```python
from build123d import *

# Parameters (mm, degrees)
SKETCH1_W               = 100
SKETCH1_H               = 65
BOSS_EXTRUDE1_DEPTH     = 75
SKETCH5_W               = 41
SKETCH5_H               = 10
CUT_EXTRUDE1_DEPTH      = 141
SKETCH6_OUTSIDE_W       = 130.178
SKETCH6_OUTSIDE_H       = 95.178
SKETCH6_OUTSIDE_W_2     = 100
SKETCH6_OUTSIDE_H_2     = 40
CUT_EXTRUDE2_DEPTH      = 1
CUT_EXTRUDE2_DEPTH_BACK = 50
SKETCH7_W               = 50
SKETCH7_H               = 20
CUT_EXTRUDE3_DEPTH      = 40
SKETCH10_W              = 40
SKETCH10_H              = 25
CUT_EXTRUDE4_DEPTH      = 40


with BuildPart() as part:
    # Sketch1 → Boss-Extrude1 (new body)
    with BuildSketch(Plane(origin=(0, 0, 0), x_dir=(1, 0, 0), z_dir=(0, 1, 0))):
        with Locations((-6.156156156, 9.992492492)):
            Rectangle(SKETCH1_W, SKETCH1_H)
    extrude(amount=BOSS_EXTRUDE1_DEPTH)

    # Sketch5 → Cut-Extrude1 (cut)
    with BuildSketch(Plane(origin=(43.843843844, 0, 0), x_dir=(0, 0, -1), z_dir=(1, 0, 0))):
        with Locations((9.992492492, 5)):
            Rectangle(SKETCH5_W, SKETCH5_H)
    extrude(amount=-CUT_EXTRUDE1_DEPTH, mode=Mode.SUBTRACT)

    # Sketch6 outside → Cut-Extrude2 (cut, two sides)
    with BuildSketch(Plane(origin=(0, 75, 0), x_dir=(1, 0, 0), z_dir=(0, 1, 0))) as cut_extrude2_sk:
        with Locations((-6.156, 9.992)):
            Rectangle(SKETCH6_OUTSIDE_W, SKETCH6_OUTSIDE_H)
        with Locations((-6.156156156, 22.492492492)):
            Rectangle(SKETCH6_OUTSIDE_W_2, SKETCH6_OUTSIDE_H_2, mode=Mode.SUBTRACT)
    extrude(amount=CUT_EXTRUDE2_DEPTH, mode=Mode.SUBTRACT)
    extrude(cut_extrude2_sk.sketch, amount=-CUT_EXTRUDE2_DEPTH_BACK, mode=Mode.SUBTRACT)

    # Sketch7 → Cut-Extrude3 (cut)
    with BuildSketch(Plane(origin=(0, 75, 0), x_dir=(1, 0, 0), z_dir=(0, 1, 0))):
        with Locations((-6.156156156, 12.492492492)):
            Rectangle(SKETCH7_W, SKETCH7_H)
    extrude(amount=-CUT_EXTRUDE3_DEPTH, mode=Mode.SUBTRACT)

    # Sketch10 → Cut-Extrude4 (cut)
    with BuildSketch(Plane(origin=(0, 25, 0), x_dir=(1, 0, 0), z_dir=(0, 1, 0))):
        with Locations((-6.156156156, -10.007507508)):
            Rectangle(SKETCH10_W, SKETCH10_H)
    extrude(amount=-CUT_EXTRUDE4_DEPTH, mode=Mode.SUBTRACT)


solid = part.part
```
The listing builds one solid part. Answer for the finished solid, in the listing's coordinates (mm). A direction names the side the tool comes from. Give positions to 0.01 mm unless a question says otherwise; leave off trailing zeros. Order: outer loops, then holes, each group sorted by start corner. A loop starts at its lowest first (then second) coordinate and runs counter-clockwise, first axis right, second up. Notation, with made-up numbers: M 78.25,-6 L 125.25,-6 A33 cw 125.25,28 Z; hole C -33.5,-0.75 d2. An arc over 180 degrees is marked long. Put each result on its own line as item: value. Start each with the question number.
Item 1: For a pull along X with two mould halves and no side action, classify faces 1 (the face through (-7, 29, -2.492)), 2 (the face through (-56.156, 37, -17)), 3 (the face through (29, 5, 10.508)) as +X half, -X half, draft (parallel to the pull), parting line (faces both ways), or undercut.
Item 2: Which of the six approach directions +Z, -Z, +X, -X, +Y, -Y give full straight-line access (tool end or side, diameter ignored) to faces 4 (the face through (-5, 5, -30.492)), 5 (the face through (-41, 0, 16)), 6 (the face through (-7, 55, -22.492)), 7 (the face through (29, 25, 10))?
Item 3: The part is cut by section B-B, the plane z = 14.5. Determine the outline of the cut face in (x, y), and give its area (3 significant figures).
Item 4: Find the intervals of material crossed by line 1 along X through (y, z) = (38, -3); line 2 along X through (y, z) = (17.5, 1.5); line 3 along Y through (x, z) = (-17, -13.5), in increasing order.
Item 5: The part is cut by section C-C, the plane x = -44. Determine the outline of the cut face in (y, z), and give its area (4 significant figures).
Item 6: The part is cut by section A-A, the plane y = 8.5. Determine the outline of the cut face in (x, z), and give its area (3 significant figures).
Item 7: Flat-ended cylindrical pins translate along their axes: P1, Ø5, axis at x = 16.5, z = -18, coming from the -Y side; P2, Ø12.5, axis at x = -46, z = 5, coming from the +Y side. Find the tip coordinate at first contact, or state that the pin passes through.
Item 8: The part is cut by section D-D, the plane y = 23. Determine the outline of the cut face in (x, z).
Answer key:
1. face 1: undercut
1. face 2: -X half
1. face 3: draft
2. face 4: +X, -X, -Y
2. face 5: +Z, -Z, +X, -X, -Y
2. face 6: +Z, +Y
2. face 7: +Z, +X, -X, +Y
3. outline: M -56.16,0 L -26.16,0 L -26.16,25 L -56.16,25 Z; M 13.84,0 L 43.84,0 L 43.84,25 L 13.84,25 Z
3. area: 1,500 mm²
4. line 1: x = -56.16 to -31.16, 18.84 to 43.84
4. line 2: x = -56.16 to -26.16, 13.84 to 43.84
4. line 3: y = 10 to 35
5. outline: M 0,-42.49 L 75,-42.49 L 75,-2.49 L 25,-2.49 L 25,22.51 L 0,22.51 L 0,10.51 L 10,10.51 L 10,-30.49 L 0,-30.49 Z
5. area: 3,215 mm²
6. outline: M -56.16,-42.49 L 43.84,-42.49 L 43.84,-30.49 L -56.16,-30.49 Z; M -56.16,10.51 L -26.16,10.51 L -26.16,22.51 L -56.16,22.51 Z; M 13.84,10.51 L 43.84,10.51 L 43.84,22.51 L 13.84,22.51 Z
6. area: 1,920 mm²
7. P1: stops at y = 10
7. P2: stops at y = 25
8. outline: M -56.16,-42.49 L 43.84,-42.49 L 43.84,22.51 L 13.84,22.51 L 13.84,-2.49 L -26.16,-2.49 L -26.16,22.51 L -56.16,22.51 Z
